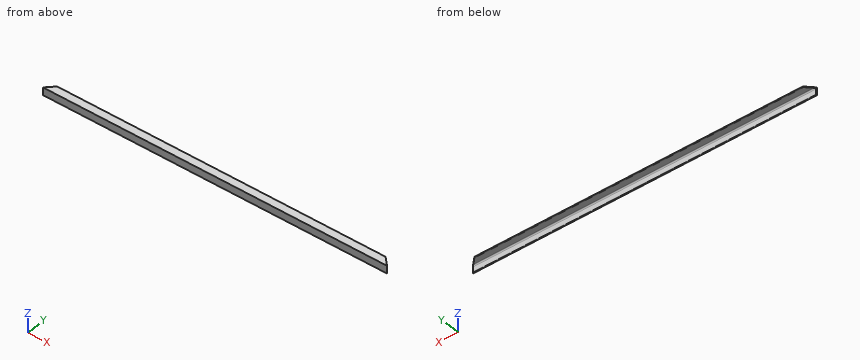
```python
from build123d import *

# Parameters (mm, degrees)
L_ANGLE_EQUAL_40X40X3_7_DEPTH = 1760
CUT_EXTRUDE1_DEPTH            = 1761.908856244


with BuildPart() as part:
    # Sketch13 → L angle (equal) 40X40X3(7) (new body)
    with BuildSketch(Plane(origin=(0, 0, 0), x_dir=(0, 0, -1), z_dir=(1, 0, 0))):
        with BuildLine():
            Line((0, 40), (0, 0))
            Line((0, 0), (40, 0))
            ThreePointArc((40, 0), (39.121320344, 2.121320344), (37, 3))
            Line((37, 3), (9, 3))
            ThreePointArc((9, 3), (4.757359313, 4.757359313), (3, 9))
            Line((3, 9), (3, 37))
            ThreePointArc((3, 37), (2.121320344, 39.121320344), (0, 40))
        make_face()
    extrude(amount=L_ANGLE_EQUAL_40X40X3_7_DEPTH)

    # Sketch14 → Cut-Extrude1 (cut, through all)
    with BuildSketch(Plane.XY):
        Polygon((1760, 0), (1760, 40), (1720, 40), align=None)
        Polygon((0, 40), (0, 0), (40, 40), align=None)
    extrude(amount=-CUT_EXTRUDE1_DEPTH, mode=Mode.SUBTRACT)


solid = part.part
```
Part model, mm, in its own coordinate system. Round coordinates to 2 decimals unless told otherwise and drop trailing zeros. Write each loop counter-clockwise with the first axis right and the second up, starting at its lowest first coordinate (ties: lowest second). Pieces come first, ordered by that corner, then holes.
Item 1: Probe L1, parallel to Z at x = 1038, y = 37.5; L2, parallel to Y at x = 1410.5, z = -24; L3, parallel to X at y = 12, z = -1.5. List the from-to ranges inside material, lowest first.
Results:
L1: z = -2.96 to 0
L2: y = 0 to 3
L3: x = 12 to 1748
Item 2: Cut at C-C, the plane y = 17. Give the cut face in (x, z).
Results:
outline: (17, -3) - (1743, -3) - (1743, 0) - (17, 0) - close
Item 3: Drop flat-ended pins along their axis: pin 1 Ø8.5 at (x, y) = (1250, 26) entering from -Z; pin 2 Ø8.5 at (x, z) = (893, -24.5) entering from +Y. Give the stop position or say it passes through.
Results:
pin 1: stops at z = -3
pin 2: stops at y = 3
Item 4: Cut at B-B, the plane z = -20. Give the cut face in (x, y), plus the area to 3 significant figures.
Results:
outline: (0, 0) - (1760, 0) - (1757, 3) - (3, 3) - close
area: 5,270 mm2
Item 5: Cut at A-A, the plane x = 915. Give the cut face in (y, z), plus the area to 3 significant figures.
Results:
outline: (0, -40) arc R3 ccw to (3, -37) - (3, -9) arc R6 cw to (9, -3) - (37, -3) arc R3 ccw to (40, 0) - (0, 0) - close
area: 235 mm2
